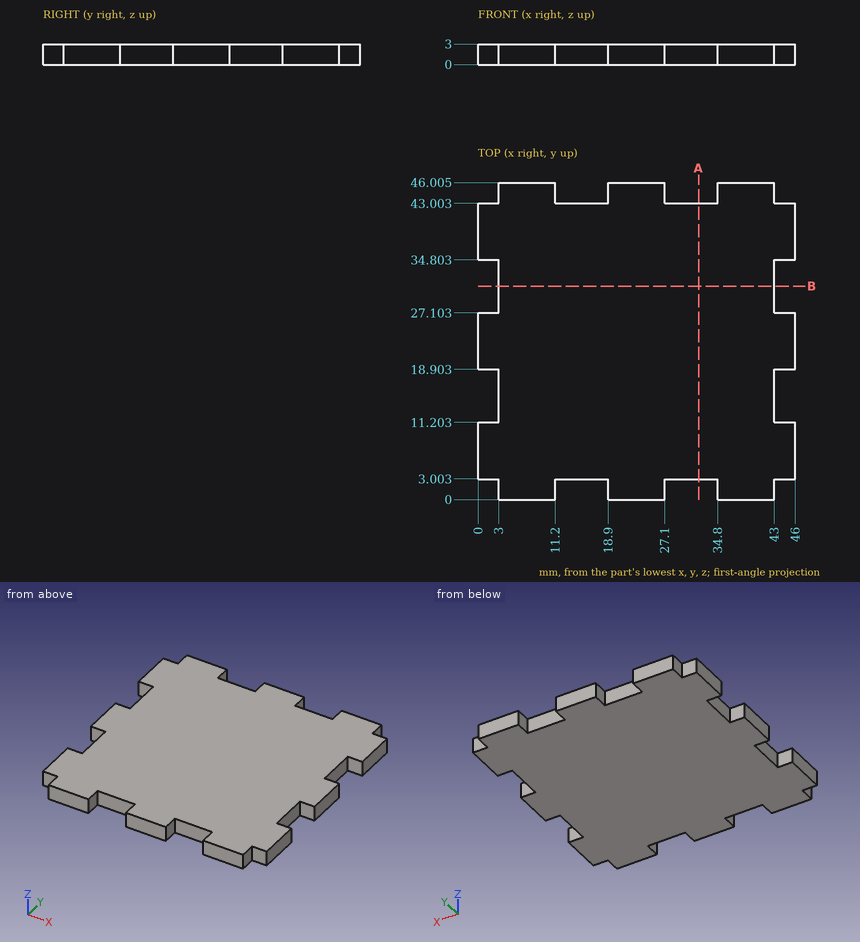
Design review of the part shown in the three views and the two pictorial views. Dimensions are in mm from the part's minimum x, y and z. Round coordinates to 2 decimals unless told otherwise and drop trailing zeros. Order: outer loops, then holes, each group sorted by start corner. A loop starts at its lowest first (then second) coordinate and runs counter-clockwise, first axis right, second up.
(1) Wall thickness on L1, parallel to X at y = 43.5, z = 0.25; L2, parallel to Y at x = 33.5, z = 1.05: over which ranges is each line inside the solid? List them lowest first.
Working result:
L1: x = 3 to 11.2, 18.9 to 27.1, 34.8 to 43
L2: y = 3 to 43
(2) Take a section at A-A, the plane x = 32. State the section outline as (y, z) points.
Working result:
outline: (3, 0) - (43, 0) - (43, 3) - (3, 3) - close
(3) For P1, Ø0.9, axis at x = 30, z = 1.5, coming from the +Y side; P2, Ø1, axis at y = 33, z = 2.5, coming from the -X side; P3, Ø0.9, axis at x = 45, z = 1, coming from the -Y side, all flat-tipped, find the tip position at first contact; note any pin that passes through.
Working result:
P1: stops at y = 43
P2: stops at x = 3
P3: stops at y = 3
